Can you work these out from the model? Positions are in its coordinate system, mm. Round coordinates to 2 decimals unless told otherwise and drop trailing zeros. Loops run counter-clockwise (first coordinate to the right, second up) from the corner with the lowest first, then second, coordinate; pieces in that order, holes last. Notation, with made-up numbers: (19, -18.5) -> (56, -18.5) arc R22 ccw to (56, 2.5) -> close; hole circle Ø10 at (52, 69.25). An arc over 180 degrees is marked (long way). Write item = value, one per line.
from build123d import *

# Parameters (mm, degrees)
ESQUISSE1_W             = 117
ESQUISSE1_H             = 10
ENL_V_MAT_EXTRU_1_REACH = 119.852
ESQUISSE2_R             = 2.5
ENL_V_MAT_EXTRU_2_REACH = 119.852
ESQUISSE3_W             = 20
ESQUISSE3_H             = 5


with BuildPart() as part:
    # Esquisse1 → Révolution1 (revolve)
    with BuildSketch(Plane.XY):
        with Locations((-58.5, 5)):
            Rectangle(ESQUISSE1_W, ESQUISSE1_H)
    revolve(axis=Axis((0, 0, 0), (-1, 0, 0)))

    # Esquisse2 → Enlèv. mat.-Extru.1 (cut, up to next)
    with BuildSketch(Plane(origin=(0, 0, 0), x_dir=(0, 0, -1), z_dir=(1, 0, 0)), mode=Mode.PRIVATE) as enl_v_mat_extru_1_sk1:
        with Locations(Location((0, 0, 0), (0, 0, 90))):
            Circle(ESQUISSE2_R)
    enl_v_mat_extru_1_tool1 = extrude(enl_v_mat_extru_1_sk1.sketch, amount=-ENL_V_MAT_EXTRU_1_REACH, mode=Mode.PRIVATE) & part.part
    add(enl_v_mat_extru_1_tool1.solids().sort_by_distance((0, 0, 0))[0], mode=Mode.SUBTRACT)

    # Esquisse3 → Enlèv. mat.-Extru.2 (cut, up to next)
    with BuildSketch(Plane(origin=(0, 0, 0), x_dir=(0, 0, -1), z_dir=(1, 0, 0)), mode=Mode.PRIVATE) as enl_v_mat_extru_2_sk1:
        with Locations((0, 7.5)):
            Rectangle(ESQUISSE3_W, ESQUISSE3_H)
    enl_v_mat_extru_2_tool1 = extrude(enl_v_mat_extru_2_sk1.sketch, amount=-ENL_V_MAT_EXTRU_2_REACH, mode=Mode.PRIVATE) & part.part
    add(enl_v_mat_extru_2_tool1.solids().sort_by_distance((0, 7.5, 0))[0], mode=Mode.SUBTRACT)


solid = part.part
1. I need wall thicknesses on line 1 (Z direction, x = -27.5, y = 0); line 2 (Y direction, x = -86, z = -1.25); line 3 (Z direction, x = -91.5, y = -1.25). Which ranges of each line are inside material? Lowest first, please. Write a range as [from, to].
Entries:
line_1 = [-10, -2.5], [2.5, 10]
line_2 = [-9.92, -2.17], [2.17, 5]
line_3 = [-9.92, -2.17], [2.17, 9.92]
2. We'd pull the mould along Y, two halves only. Please class faces 1 (the cylindrical face through (-58, -10, 0)), 2 (the flat face through (0, -2, 2)), 3 (the flat face through (-58, 5, 0)), 4 (the cylindrical face through (-57.68, -0.54, -2.44)): released by +Y, released by -Y, zero draft, split by the parting line, or undercut.
Entries:
face_1 = split by the parting line
face_2 = zero draft
face_3 = released by +Y
face_4 = undercut
3. Suppose I cut it at D-D, the plane y = -8. List the corners of the cut face in (x, z) for me.
Entries:
outline = (-117, -6) -> (0, -6) -> (0, 6) -> (-117, 6) -> close
4. Suppose I cut it at B-B, the plane z = 0. List the corners of the cut face in (x, y) for me, and give its area (3 significant figures).
Entries:
outline = (-117, -10) -> (0, -10) -> (0, -2.5) -> (-117, -2.5) -> close; (-117, 2.5) -> (0, 2.5) -> (0, 5) -> (-117, 5) -> close
area = 1,170 mm²
5. Suppose I cut it at A-A, the plane y = 0. List the corners of the cut face in (x, z) for me, and give its area (4 significant figures).
Entries:
outline = (-117, -10) -> (0, -10) -> (0, -2.5) -> (-117, -2.5) -> close; (-117, 2.5) -> (0, 2.5) -> (0, 10) -> (-117, 10) -> close
area = 1,755 mm²
6. Suppose I cut it at C-C, the plane x = -82. List the corners of the cut face in (y, z) for me, and give its area (3 significant figures).
Entries:
outline = (5, -8.66) -> (5, 8.66) arc R10 ccw (long way) to start; hole circle Ø5 at (0, 0)
area = 233 mm²
